```python
from build123d import *

# Parameters (mm, degrees)
SKETCH1_R           = 28.575
BOSS_EXTRUDE1_DEPTH = 9.525
CUT_EXTRUDE1_DEPTH  = 9.525
CIRPATTERN1_COUNT   = 12
SKETCH3_R           = 30.1625
BOSS_EXTRUDE2_DEPTH = 1.5875


with BuildPart() as part:
    # Sketch1 → Boss-Extrude1 (new, symmetric)
    with BuildSketch(Plane.XY):
        with Locations(Location((0, 0, 0), (0, 0, 180))):
            Circle(SKETCH1_R)
    extrude(amount=BOSS_EXTRUDE1_DEPTH, both=True)

    # Sketch2 → Cut-Extrude1 (cut, symmetric)
    with BuildSketch(Plane.XY):
        with BuildLine():
            Line((-1.5875, 28.5308687), (-1.5875, 25.3558687))
            Line((-1.5875, 25.3558687), (-4.7625, 25.3558687))
            Line((-4.7625, 25.3558687), (-4.7625, 23.7683687))
            Line((-4.7625, 23.7683687), (4.7625, 23.7683687))
            Line((4.7625, 23.7683687), (4.7625, 25.3558687))
            Line((4.7625, 25.3558687), (1.5875, 25.3558687))
            Line((1.5875, 25.3558687), (1.5875, 28.5308687))
            ThreePointArc((1.5875, 28.5308687), (0, 28.575), (-1.5875, 28.5308687))
        make_face()
    cut_extrude1 = extrude(amount=CUT_EXTRUDE1_DEPTH, both=True, mode=Mode.SUBTRACT)

    # CirPattern1: Cut-Extrude1 ×12 about axis
    cirpattern1_axis = Axis((0, 0, 0), (0, 0, 1))
    for i in range(1, CIRPATTERN1_COUNT):
        add(cut_extrude1.rotate(cirpattern1_axis, i * 360 / CIRPATTERN1_COUNT), mode=Mode.SUBTRACT)

    # Sketch3 → Boss-Extrude2 (add)
    with BuildSketch(Plane(origin=(0, 0, -9.525), x_dir=(-1, 0, 0), z_dir=(0, 0, -1))):
        Circle(SKETCH3_R)
    boss_extrude2 = extrude(amount=BOSS_EXTRUDE2_DEPTH)

    # Mirror1: Boss-Extrude2 across plane
    add(boss_extrude2.mirror(Plane.XY))


solid = part.part
```
Design review of the part built by this model. Coordinates are the model's own, in mm. A direction names the side the tool comes from. Coordinates: 2 decimals unless noted, no trailing zeros. Order: outer loops, then holes, each group sorted by start corner. A loop starts at its lowest first (then second) coordinate and runs counter-clockwise, first axis right, second up.
1) Take a section at A-A, the plane y = 0. Give the boundary of the cut face in (x, z) (1 decimal), and give its area (3 significant figures).
2) Take a section at D-D, the plane y = 26.5. Give the boundary of the cut face in (x, z) (1 decimal), and give its area (3 significant figures).
3) For faces 1 (the flat face through (-18.9, -16.41, 0.13)), 2 (the cylindrical face through (-27.58, 7.48, 0.13)), 3 (the flat face through (-22.521, 14.835, 0.133)), list the 3-axis set-ups (+Z, -Z, +X, -X, +Y, -Y) from which the entire face can be reached by the end or side of a thin tool; tool diameter is ignored.
4) Take a section at C-C, the plane y = 10. Give the boundary of the cut face in (x, z) (1 decimal), and give its area (3 significant figures).
5) Clearance check with flat-ended pins moving along their axes: pin 1 (1.6 mm diameter, centred on x = -3.5, z = -2, fed in from -Y); pin 2 (2.5 mm diameter, centred on x = -26.5, z = 4, fed in from -Y); pin 3 (0.5 mm diameter, centred on x = -24, z = 0, fed in from -Y). State where each tip first meets the part, or that it passes through.
6) Wall thickness on line 1 along Y through (x, z) = (2, -5.25); line 2 along X through (y, z) = (-8.5, -6.25); line 3 along Y through (x, z) = (21, -4.5): over which ranges is each line inside the solid? List them lowest first.
Returned:
1. outline: (-30.2, -11.1) - (30.2, -11.1) - (30.2, -9.5) - (23.8, -9.5) - (23.8, 9.5) - (30.2, 9.5) - (30.2, 11.1) - (-30.2, 11.1) - (-30.2, 9.5) - (-23.8, 9.5) - (-23.8, -9.5) - (-30.2, -9.5) - close
1. area: 1,100 mm2
2. outline: (-14.4, -11.1) - (14.4, -11.1) - (14.4, -9.5) - (10.7, -9.5) - (10.7, 9.5) - (14.4, 9.5) - (14.4, 11.1) - (-14.4, 11.1) - (-14.4, 9.5) - (-10.7, 9.5) - (-10.7, -9.5) - (-14.4, -9.5) - close; hole (-1.6, -9.5) - (1.6, -9.5) - (1.6, 9.5) - (-1.6, 9.5) - close
2. area: 438 mm2
3. face 1: none
3. face 2: -X, +Y
3. face 3: -X
4. outline: (-28.5, -11.1) - (28.5, -11.1) - (28.5, -9.5) - (26.8, -9.5) - (26.8, 9.5) - (28.5, 9.5) - (28.5, 11.1) - (-28.5, 11.1) - (-28.5, 9.5) - (-26.8, 9.5) - (-26.8, -9.5) - (-28.5, -9.5) - close; hole (-23.5, -9.5) - (-21.7, -9.5) - (-21.7, 9.5) - (-23.5, 9.5) - close; hole (21.7, -9.5) - (23.5, -9.5) - (23.5, 9.5) - (21.7, 9.5) - close
4. area: 1,130 mm2
5. pin 1: stops at y = -28.45
5. pin 2: stops at y = -12.89
5. pin 3: stops at y = -15.89
6. line 1: y = -28.5 to -25.36, -23.77 to 23.77, 25.36 to 28.5
6. line 2: x = -27.28 to -24.25, -22.54 to 22.54, 24.25 to 27.28
6. line 3: y = -19.38 to -14.34, -11.16 to 11.16, 14.34 to 19.38
